```python
from build123d import *

# Parameters (mm, degrees)
F0_R     = 2
F1_DEPTH = 5


# Not quite as in the source:
# - a feature names something its author has since deleted; it is built from what else it names


with BuildPart() as f1:
    # F0 (on Front) → F1 (new body)
    with BuildSketch(Plane.XZ):
        Polygon((-8.8270233517, 0), (-36.085901234, 0), (-36.085901234, -4), (0, -4), (0, 0), (-15.2059999965, 32.6093722259), (-22.4564622928, 29.2284261319), align=None)
        with Locations((-6.4696469888, 4.4093964081)):
            Circle(F0_R, mode=Mode.SUBTRACT)
        Polygon((-36.085901234, 58.4568522639), (-22.4564622928, 29.2284261319), (-15.2059999965, 32.6093722259), (-28.8354389377, 61.8377983578), align=None)
        with Locations((-31.1928153006, 57.4284019497)):
            Circle(F0_R, mode=Mode.SUBTRACT)
    extrude(amount=F1_DEPTH)


solid = f1.part
```
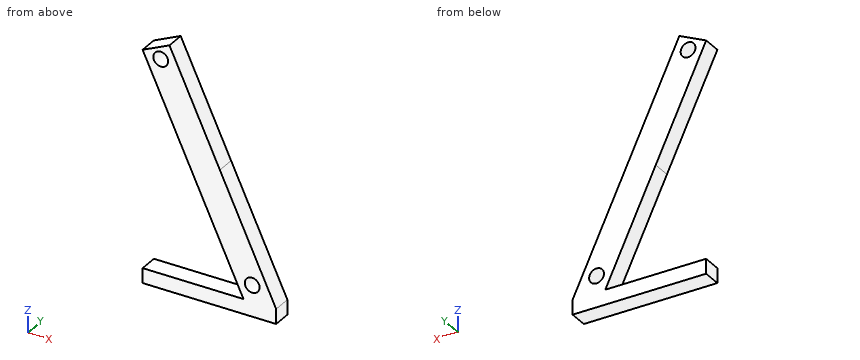
CAD build for the part. Positions are in the model's coordinates, mm. Round coordinates to 2 decimals unless told otherwise and drop trailing zeros. Order: outer loops, then holes, each group sorted by start corner. A loop starts at its lowest first (then second) coordinate and runs counter-clockwise, first axis right, second up. Notation, with made-up numbers: (50, 46) - (58, 46) arc R9 ccw to (58, 57) - close; hole circle Ø5 at (68, 78.25). An arc over 180 degrees is marked (long way). Answer as CSV lines item,"result". Start each with the question number.
1. Drill centre lines: L1, parallel to Z at x = -31, y = -0.45; L2, parallel to Z at x = -27, y = -2.1; L3, parallel to Z at x = -28.5, y = -4.55. Where is each one in solid material? Low to high. Write a range as [from, to].
2. Pin check, flat tips, straight feed: pin 1 (1.5 mm diameter, centred on y = -2, z = 29.5, fed in from +X); pin 2 (8 mm diameter, centred on x = -16.5, z = 42, fed in from +Y). Stop position of each tip, or through.
3. Saw through at B-B, the plane y = -0.85. Write the cut outline in (x, z), and give its area (3 significant figures).
4. Saw through at D-D, the plane x = -2.5. Write the cut outline in (y, z).
5. Saw through at C-C, the plane z = 34. Write the cut outline in (x, y).
6. Saw through at A-A, the plane x = -12. Write the cut outline in (y, z).
Model answer:
1,L1,"z = [-4, 0], [47.55, 55.44], [59.42, 60.83]"
1,L2,"z = [-4, 0], [38.97, 57.9]"
1,L3,"z = [-4, 0], [42.19, 61.12]"
2,pin 1,"stops at x = -13.41"
2,pin 2,"stops at y = 0"
3,outline,"(-36.09, -4) - (0, -4) - (0, 0) - (-28.84, 61.84) - (-36.09, 58.46) - (-8.83, 0) - (-36.09, 0) - close; hole circle Ø4 at (-31.19, 57.43); hole circle Ø4 at (-6.47, 4.41)"
3,area,"650 mm²"
4,outline,"(-5, -4) - (0, -4) - (0, 5.36) - (-5, 5.36) - close"
5,outline,"(-24.68, -5) - (-15.85, -5) - (-15.85, 0) - (-24.68, 0) - close"
6,outline,"(-5, -4) - (0, -4) - (0, 0) - (-5, 0) - close; (-5, 6.8) - (0, 6.8) - (0, 25.73) - (-5, 25.73) - close"
